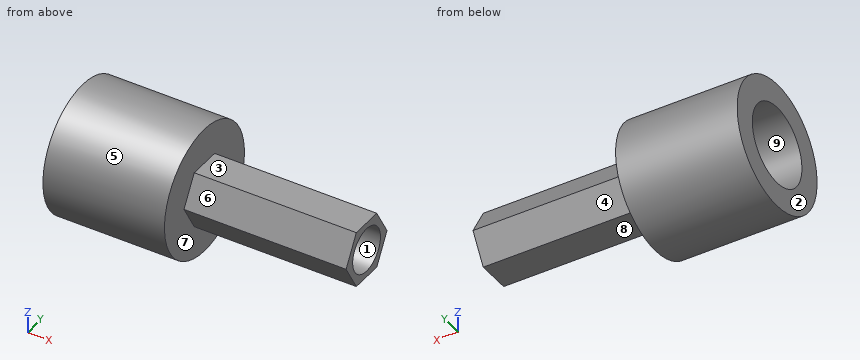
from build123d import *

# Parameters (mm, degrees)
SALIENTE_EXTRUIR1_DEPTH = 20
CROQUIS2_R              = 7.9
CROQUIS2_R_2            = 4.9
SALIENTE_EXTRUIR2_DEPTH = 3
SALIENTE_EXTRUIR3_START = 3
CROQUIS2_3_R            = 7.9
CROQUIS2_3_R_2          = 4.9
SALIENTE_EXTRUIR3_DEPTH = 12
CROQUIS3_R              = 2.75
CORTAR_EXTRUIR1_DEPTH   = 37.73989657
CROQUIS5_R              = 2.75
SALIENTE_EXTRUIR4_DEPTH = 0.3


with BuildPart() as part:
    # Croquis1 → Saliente-Extruir1 (new body)
    with BuildSketch(Plane(origin=(0, 0, 0), x_dir=(0, 0, -1), z_dir=(1, 0, 0))):
        Polygon((-3.5, -2.020725942), (0, -4.041451884), (3.5, -2.020725942), (3.5, 2.020725942), (0, 4.041451884), (-3.5, 2.020725942), align=None)
    extrude(amount=SALIENTE_EXTRUIR1_DEPTH)

    # Croquis2 → Saliente-Extruir2 (add)
    with BuildSketch(Plane.ZY):
        Circle(CROQUIS2_R)
        Circle(CROQUIS2_R_2, mode=Mode.SUBTRACT)
        Circle(CROQUIS2_R_2)
        Polygon((3.5, -2.020725942), (3.5, 2.020725942), (0, 4.041451884), (-3.5, 2.020725942), (-3.5, -2.020725942), (0, -4.041451884), align=None, mode=Mode.SUBTRACT)
        Polygon((0, -4.041451884), (3.5, -2.020725942), (3.5, 2.020725942), (0, 4.041451884), (-3.5, 2.020725942), (-3.5, -2.020725942), align=None)
    extrude(amount=SALIENTE_EXTRUIR2_DEPTH)

    # Croquis2<3> → Saliente-Extruir3 (add)
    with BuildSketch(Plane.ZY.offset(SALIENTE_EXTRUIR3_START)):
        Circle(CROQUIS2_3_R)
        Circle(CROQUIS2_3_R_2, mode=Mode.SUBTRACT)
    extrude(amount=SALIENTE_EXTRUIR3_DEPTH)

    # Croquis3 → Cortar-Extruir1 (cut, through all)
    with BuildSketch(Plane(origin=(20, 0, 0), x_dir=(0, 0, -1), z_dir=(1, 0, 0))):
        Circle(CROQUIS3_R)
    extrude(amount=-CORTAR_EXTRUIR1_DEPTH, mode=Mode.SUBTRACT)

    # Croquis5 → Saliente-Extruir4 (add)
    with BuildSketch(Plane.ZY.offset(3)):
        with Locations(Location((0, 0, 0), (0, 0, 180))):
            Circle(CROQUIS5_R)
    extrude(amount=-SALIENTE_EXTRUIR4_DEPTH)


solid = part.part
Work out the finished part from the listing and answer in its coordinate system (mm). Face numbers are marked on the shaded views. A direction names the side the tool comes from. Round coordinates to 2 decimals unless told otherwise and drop trailing zeros. Write each loop counter-clockwise with the first axis right and the second up, starting at its lowest first coordinate (ties: lowest second). Pieces come first, ordered by that corner, then holes. Notation, with made-up numbers: (58.25, 39.25) - (79.25, 39.25) arc R20 cw to (79.25, 59.25) - close; hole circle Ø4 at (30, -22). An arc over 180 degrees is marked (long way). Answer in a Markdown table with one row per item. Add a question column.
1. A cutting plane is placed at B-B, the plane y = 0. Determine the outline of the cut face in (x, z).
2. The mould has two halves that part along Z. Classify the marked faces 1, 2, 3 and 4: +Z half, -Z half, draft (parallel to the pull), parting line (faces both ways), or undercut.
3. Find the intervals of material crossed by line 1 along Y through (x, z) = (-10, 0); line 2 along Z through (x, y) = (4, 0); line 3 along X through (y, z) = (2.25, 0.75), in increasing order. Write a range as from..to.
4. Given pin 1 (3 mm diameter, centred on y = 0, z = 0, fed in from +X); pin 2 (1.5 mm diameter, centred on x = 8.5, z = 3.5, fed in from +Y); pin 3 (1 mm diameter, centred on x = -10, z = -1.5, fed in from -Y), each flat-ended and moving along its own axis, determine where each tip first touches the part or whether it passes through.
5. A cutting plane is placed at D-D, the plane x = -6. Determine the outline of the cut face in (y, z), and give its area (3 significant figures).
6. A cutting plane is placed at C-C, the plane z = -4.5. Determine the outline of the cut face in (x, y).
7. For the marked faces 5, 6, 7, 8 and 9, determine the directions among +Z, -Z, +X, -X, +Y, -Y from which every point of the face is accessible in a straight line to the end or side of a thin tool.
8. A cutting plane is placed at A-A, the plane x = 8. Determine the outline of the cut face in (y, z), and give its area (3 significant figures).
Worked out:
| question | item | result |
|---|---|---|
| 1 | outline | (-15, -7.9) - (0, -7.9) - (0, -3.5) - (20, -3.5) - (20, -2.75) - (-2.7, -2.75) - (-2.7, 2.75) - (20, 2.75) - (20, 3.5) - (0, 3.5) - (0, 7.9) - (-15, 7.9) - (-15, 4.9) - (-3, 4.9) - (-3, -4.9) - (-15, -4.9) - close |
| 2 | face 1 | undercut |
| 2 | face 2 | draft |
| 2 | face 3 | +Z half |
| 2 | face 4 | -Z half |
| 3 | line 1 | -7.9..-4.9, 4.9..7.9 |
| 3 | line 2 | -3.5..-2.75, 2.75..3.5 |
| 3 | line 3 | -3..-2.7 |
| 4 | pin 1 | x = -2.7 |
| 4 | pin 2 | y = 2.45 |
| 4 | pin 3 | y = -7.84 |
| 5 | outline | circle Ø15.8 at (0, 0); hole circle Ø9.8 at (0, 0) |
| 5 | area | 121 mm^2 |
| 6 | outline | (-15, -6.49) - (0, -6.49) - (0, 6.49) - (-15, 6.49) - (-15, 1.94) - (-3, 1.94) - (-3, -1.94) - (-15, -1.94) - close |
| 7 | face 5 | +X, -X |
| 7 | face 6 | +Z, +X, -Y |
| 7 | face 7 | +X |
| 7 | face 8 | -Z, +X, +Y, -Y |
| 7 | face 9 | -X |
| 8 | outline | (-4.04, 0) - (-2.02, -3.5) - (2.02, -3.5) - (4.04, 0) - (2.02, 3.5) - (-2.02, 3.5) - close; hole circle Ø5.5 at (0, 0) |
| 8 | area | 18.7 mm^2 |
